```python
from build123d import *

# Parameters (mm, degrees)
SKETCH1_W               = 13
SKETCH1_H               = 8
BOSS_EXTRUDE1_DEPTH     = 3
CUT_EXTRUDE1_DEPTH      = 16.556349186
CUT_EXTRUDE1_DEPTH_BACK = 16.556349186
CUT_EXTRUDE2_DEPTH      = 16.556349186
CUT_EXTRUDE2_DEPTH_BACK = 16.556349186
SKETCH4_R               = 1.8
CUT_EXTRUDE3_DEPTH      = 0.8
SKETCH5_W               = 8
SKETCH5_H               = 1.1
BOSS_EXTRUDE2_DEPTH     = 2
FILLET1_R               = 4
CUT_EXTRUDE4_DEPTH      = 0.4


with BuildPart() as part:
    # Sketch1 → Boss-Extrude1 (new body)
    with BuildSketch(Plane(origin=(0, 0, 0), x_dir=(1, 0, 0), z_dir=(0, 1, 0))):
        with Locations((6.5, 4)):
            Rectangle(SKETCH1_W, SKETCH1_H)
    extrude(amount=BOSS_EXTRUDE1_DEPTH)

    # Sketch2 → Cut-Extrude1 (cut, two sides: drawn at the far end of the back side and taken through both)
    with BuildSketch(Plane.XY.offset(-CUT_EXTRUDE1_DEPTH_BACK)):
        Polygon((0, 0), (0.6, 3), (0, 3), align=None)
        Polygon((13, 0), (12.4, 3), (13, 3), align=None)
    extrude(amount=CUT_EXTRUDE1_DEPTH + CUT_EXTRUDE1_DEPTH_BACK, mode=Mode.SUBTRACT)

    # Sketch3 → Cut-Extrude2 (cut, two sides: drawn at the far end of the back side and taken through both)
    with BuildSketch(Plane(origin=(0, 0, 0), x_dir=(0, 0, -1), z_dir=(1, 0, 0)).offset(-CUT_EXTRUDE2_DEPTH_BACK)):
        Polygon((0, 0), (0.6, 3), (0, 3), align=None)
        Polygon((8, 3), (7.4, 3), (8, 0), align=None)
    extrude(amount=CUT_EXTRUDE2_DEPTH + CUT_EXTRUDE2_DEPTH_BACK, mode=Mode.SUBTRACT)

    # Sketch4 → Cut-Extrude3 (cut)
    with BuildSketch(Plane.XZ):
        with Locations(Location((6.50000125, -3.75, 0), (0, 0, 270))):
            Circle(SKETCH4_R)
    extrude(amount=-CUT_EXTRUDE3_DEPTH, mode=Mode.SUBTRACT)

    # Sketch5 → Boss-Extrude2 (add)
    with BuildSketch(Plane.XZ):
        with Locations((6.500011, -7.45)):
            Rectangle(SKETCH5_W, SKETCH5_H)
    extrude(amount=BOSS_EXTRUDE2_DEPTH)

    # Fillet1
    # the kernel refuses this fillet: 4 mm, written as the material it takes off along each edge
    with BuildSketch(Plane(origin=(10.500011, -2, -16.660254038), x_dir=(0, 1, 0), z_dir=(0, 0, 1)), Plane(origin=(2.500011, -2, 1.760254038), x_dir=(0, 1, 0), z_dir=(0, 0, -1))) as fillet1_piece_1:
        with BuildLine():
            CenterArc((4, 3.464101615), FILLET1_R, 180, 60)
            Line((0, 3.464101615), (-0.08, 3.464101615))
            Line((-0.08, 3.464101615), (-0.08, 0))
            Line((-0.08, 0), (0, -0.08))
            ThreePointArc((0, -0.08), (1, -0.08), (1.96, -0.069282032))
            Line((1.96, -0.069282032), (2, 0))
        make_face()
    extrude(amount=18.420508076, mode=Mode.SUBTRACT)

    # Sketch6 → Cut-Extrude4 (cut)
    with BuildSketch(Plane(origin=(0, 3, 0), x_dir=(1, 0, 0), z_dir=(0, 1, 0))):
        Polygon((4.028737707, 2.518536397), (4.028737707, 5.518536397), (6.067199245, 5.518536397), (6.067199245, 5.018536397), (4.605660784, 5.018536397), (4.605660784, 4.287767167), (5.874891553, 4.287767167), (5.874891553, 3.787767167), (4.605660784, 3.787767167), (4.605660784, 2.518536397), align=None)
        Polygon((6.567199245, 2.518536397), (6.567199245, 5.518536397), (7.169963668, 5.518536397), (8.374891553, 3.546180628), (8.374891553, 5.518536397), (8.95181463, 5.518536397), (8.95181463, 2.518536397), (8.330420399, 2.518536397), (7.144122322, 4.459642167), (7.144122322, 2.518536397), align=None)
    extrude(amount=-CUT_EXTRUDE4_DEPTH, mode=Mode.SUBTRACT)


solid = part.part
```
Geometry: final body of the model. Coordinates: model frame, mm. A direction names the side the tool comes from. Give positions to 0.01 mm unless a question says otherwise; leave off trailing zeros. Loops run counter-clockwise (first coordinate to the right, second up) from the corner with the lowest first, then second, coordinate; pieces in that order, holes last. Notation, with made-up numbers: (36, -37.5) -> (83, -37.5) arc R27 cw to (83, -19.5) -> close; hole circle Ø10 at (53, -14.75). An arc over 180 degrees is marked (long way). Use CSV: the item, a comma, the result in double quotes.
(1) Cut plane C-C (y = 2.25). Output: boundary loops of the cut face in (x, z).
From the geometry:
outline,"(0.45, -7.55) -> (12.55, -7.55) -> (12.55, -0.45) -> (0.45, -0.45) -> close"
(2) Ray query, line 1 along Y through (x, z) = (8, -5); line 2 along Z through (x, y) = (6.75, 2.7); line 3 along X through (y, z) = (0.65, -5). Return the intervals inside material, ascending. Write a range as [from, to].
From the geometry:
line 1,"[0, 3]"
line 2,"[-7.46, -5.52], [-2.52, -0.54]"
line 3,"[0.13, 5.2], [7.8, 12.87]"
(3) Cut plane A-A (x = 3.5). Output: boundary loops of the cut face in (y, z).
From the geometry:
outline,"(-1.15, -8) -> (0, -8) -> (3, -7.4) -> (3, -0.6) -> (0, 0) -> (0, -6.9) -> (-1.15, -6.9) -> close"
(4) Cut plane D-D (x = 2). Output: boundary loops of the cut face in (y, z).
From the geometry:
outline,"(0, -8) -> (3, -7.4) -> (3, -0.6) -> (0, 0) -> close"
(5) Access query for faces 5 (the face through (7.746, 2.803, -3.476)), 6 (the face through (7, 0.8, -4)), 7 (the face through (12.7, 1.5, -4.1)). Directions: +Z, -Z, +X, -X, +Y, -Y. A direction counts if a zero-diameter tool reaches every point of the face in a straight line with its end or side. Return the directions, or none.
From the geometry:
face 5,"+Y"
face 6,"-Y"
face 7,"+Z, -Z, +X, +Y"
(6) Cut plane B-B (z = -4). Output: boundary loops of the cut face in (x, y).
From the geometry:
outline,"(0, 0) -> (4.72, 0) -> (4.72, 0.8) -> (8.28, 0.8) -> (8.28, 0) -> (13, 0) -> (12.4, 3) -> (8.95, 3) -> (8.95, 2.6) -> (8.37, 2.6) -> (8.37, 3) -> (8.1, 3) -> (8.1, 2.6) -> (7.43, 2.6) -> (7.43, 3) -> (7.14, 3) -> (7.14, 2.6) -> (6.57, 2.6) -> (6.57, 3) -> (5.87, 3) -> (5.87, 2.6) -> (4.03, 2.6) -> (4.03, 3) -> (0.6, 3) -> close"
(7) Pull-direction query (Z, two-part tool) for faces 1 (the face through (6, -1, -6.9)), 2 (the face through (6.4, 1.5, -7.7)), 3 (the face through (5.811, 0.394, -5.413)), 4 (the face through (6.5, -2, -7.4)); classes: released by +Z, released by -Z, zero draft, split by the parting line, or undercut.
From the geometry:
face 1,"released by +Z"
face 2,"released by -Z"
face 3,"undercut"
face 4,"zero draft"
(8) First-contact query: P1, Ø4, axis at x = 5.5, z = -3.5, coming from the -Y side; P2, Ø2, axis at y = 2, z = -3.5, coming from the +X side; P3, Ø3, axis at x = 6.5, z = -3.75, coming from the -Y side. Flat tips, straight axial feed; report the tip coordinate or a pass-through.
From the geometry:
P1,"y = 0"
P2,"x = 12.8"
P3,"y = 0.8"
